Geometry check sheet. Reference: the model listing, model coordinates, mm. Face numbers are marked on the shaded views. A direction names the side the tool comes from. Coordinates: 2 decimals unless noted, no trailing zeros. Write each loop counter-clockwise with the first axis right and the second up, starting at its lowest first coordinate (ties: lowest second). Pieces come first, ordered by that corner, then holes. Notation, with made-up numbers: M 63.5,62.25 L 107.5,62.25 A23 cw 107.5,98.25 Z; hole C -37.5,16 d7. An arc over 180 degrees is marked long. Answer as a JSON object with one key per item and string values. Group by question number.
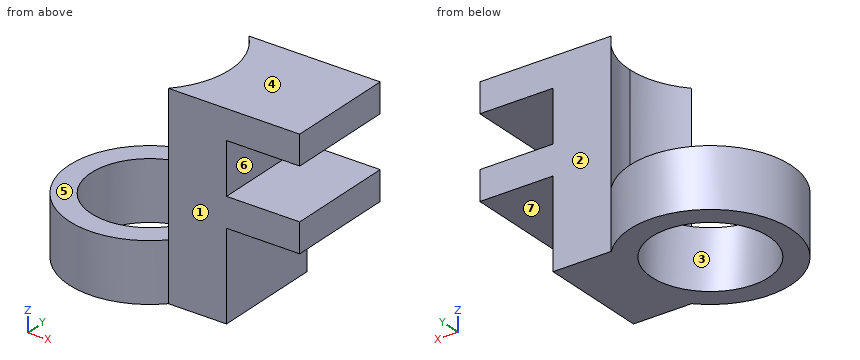
```python
from build123d import *

# Parameters (mm, degrees)
F0_R     = 8
F1_DEPTH = 8
F2_DEPTH = 27
F3_W     = 15
F3_H     = 4
F4_DEPTH = 10
F5_W     = 15
F5_H     = 4
F6_DEPTH = 10


with BuildPart() as f1:
    # F0 (on Top) → F1 (new body)
    with BuildSketch(Plane.XY):
        Circle(F0_R)
        with BuildLine():
            ThreePointArc((8.046738, -7.5), (10.23509, -4.030253), (11, 0))
            ThreePointArc((11, 0), (10.23509, 4.030253), (8.046738, 7.5))
            ThreePointArc((8.046738, 7.5), (-11, 0), (8.046738, -7.5))
        make_face()
        Circle(F0_R, mode=Mode.SUBTRACT)
        with BuildLine():
            ThreePointArc((8.046738, 7.5), (10.23509, 4.030253), (11, 0))
            Line((11, 0), (16, 0))
            Line((16, 0), (16, 7.5))
            Line((16, 7.5), (8.046738, 7.5))
        make_face()
        with BuildLine():
            Line((16, 0), (11, 0))
            ThreePointArc((11, 0), (10.23509, -4.030253), (8.046738, -7.5))
            Line((8.046738, -7.5), (16, -7.5))
            Line((16, -7.5), (16, 0))
        make_face()
    extrude(amount=F1_DEPTH)

    # F0 (on Top) → F2 (join)
    with BuildSketch(Plane.XY):
        with BuildLine():
            ThreePointArc((8.046738, 7.5), (10.23509, 4.030253), (11, 0))
            Line((11, 0), (16, 0))
            Line((16, 0), (16, 7.5))
            Line((16, 7.5), (8.046738, 7.5))
        make_face()
        with BuildLine():
            Line((16, 0), (11, 0))
            ThreePointArc((11, 0), (10.23509, -4.030253), (8.046738, -7.5))
            Line((8.046738, -7.5), (16, -7.5))
            Line((16, -7.5), (16, 0))
        make_face()
    extrude(amount=F2_DEPTH)

    # F3 (on face) → F4 (join)
    with BuildSketch(Plane.YZ.offset(16)):
        with Locations((0, 25)):
            Rectangle(F3_W, F3_H)
    extrude(amount=F4_DEPTH)

    # F5 (on face) → F6 (join)
    with BuildSketch(Plane.YZ.offset(16)):
        with Locations((0, 14)):
            Rectangle(F5_W, F5_H)
    extrude(amount=F6_DEPTH)


solid = f1.part
```
1) Section check C-C (z = 20). Record the cut outline in (x, y).
2) Material ranges on probe 1 along Y at (x, z) = (0, 6.25); probe 2 along Y at (x, z) = (24, 24); probe 3 along Z at (x, y) = (6, -8.5), recorded low to high. Write a range as [from, to].
3) Section check A-A (x = 0). Record the cut outline in (y, z).
4) Draft check along Y on the marked faces 1, 2, 3 and 4. Enter one of: +Y half, -Y half, draft (parallel to the pull), parting line (faces both ways), or undercut.
5) Go/stop test with flat-tipped pins: pin 1 Ø4 at (x, z) = (10.5, 14.5) entering from -Y; pin 2 Ø1 at (x, z) = (-4, 6.5) entering from +Y; pin 3 Ø5 at (x, y) = (19.5, -3.5) entering from -Z; pin 4 Ø3 at (x, y) = (-5.5, -0.5) entering from -Z. Record where each tip stops, or that it passes through.
6) Section check B-B (y = -0.75). Record the cut outline in (x, z), then the cut area to 3 significant figures.
7) Set-up check for the marked faces 5, 6 and 7: record each of +Z, -Z, +X, -X, +Y, -Y from which the full face is reachable in a straight line by a thin tool's end or side.
8) Section check D-D (y = 2). Record the cut outline in (x, z).
Entries:
{
 "1": {"outline": "M 8.05,-7.5 L 16,-7.5 L 16,7.5 L 8.05,7.5 A11 cw 11,0 A11 cw Z"},
 "2": {"probe 1": "[-11, -8], [8, 11]", "probe 2": "[-7.5, 7.5]", "probe 3": "[0, 8]"},
 "3": {"outline": "M -11,0 L -8,0 L -8,8 L -11,8 Z; M 8,0 L 11,0 L 11,8 L 8,8 Z"},
 "4": {"face 1": "-Y half", "face 2": "+Y half", "face 3": "undercut", "face 4": "draft"},
 "5": {"pin 1": "y = -7.5", "pin 2": "y = 10.43", "pin 3": "z = 12", "pin 4": "through"},
 "6": {"outline": "M -10.97,0 L -7.96,0 L -7.96,8 L -10.97,8 Z; M 7.96,0 L 16,0 L 16,12 L 26,12 L 26,16 L 16,16 L 16,23 L 26,23 L 26,27 L 10.97,27 L 10.97,8 L 7.96,8 Z", "area": "264 mm^2"},
 "7": {"face 5": "+Z, -X", "face 6": "+X, +Y, -Y", "face 7": "-Z, +X, +Y, -Y"},
 "8": {"outline": "M -10.82,0 L -7.75,0 L -7.75,8 L -10.82,8 Z; M 7.75,0 L 16,0 L 16,12 L 26,12 L 26,16 L 16,16 L 16,23 L 26,23 L 26,27 L 10.82,27 L 10.82,8 L 7.75,8 Z"}
}
